```python
from build123d import *

# Parameters (mm, degrees)
RECORD_R             = 67.31
RECORD_R_2           = 1.054294776
RECORD_EXTRUDE_DEPTH = 2.54
MOTOR_HOLE_DEPTH     = 2.54


# Read off the part's stored shape, not the designer's step: Motor Hole
with BuildPart() as part:
    # Record → Record Extrude (new body)
    with BuildSketch(Plane(origin=(0, 0, 0), x_dir=(1, 0, 0), z_dir=(0, 1, 0))):
        with Locations(Location((13.743289035, -70.841587708, 0), (0, 0, 270))):
            Circle(RECORD_R)
        with Locations(Location((66.372058646, -74.952013208, 0), (0, 0, 270))):
            Circle(RECORD_R_2, mode=Mode.SUBTRACT)
        with Locations(Location((40.779568941, -74.952013208, 0), (0, 0, 270))):
            Circle(RECORD_R_2, mode=Mode.SUBTRACT)
    extrude(amount=RECORD_EXTRUDE_DEPTH)

    # Motor Hole outline → Motor Hole (cut)
    with BuildSketch(Plane(origin=(0, 0, 0), x_dir=(1, 0, 0), z_dir=(0, 1, 0))):
        with BuildLine():
            Line((11.872460342, -72.091587708), (15.614117728, -72.091587708))
            ThreePointArc((15.614117728, -72.091587708), (13.743289035, -68.591587708), (11.872460342, -72.091587708))
        make_face()
    extrude(amount=MOTOR_HOLE_DEPTH, mode=Mode.SUBTRACT)


solid = part.part
```
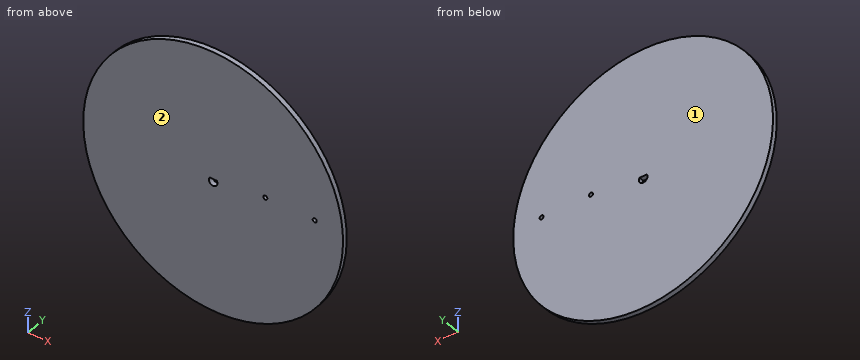
The model under review builds one solid part; all positions refer to its coordinate system, in mm. Face numbers are marked on the shaded views. Round coordinates to 2 decimals unless told otherwise and drop trailing zeros. Order: outer loops, then holes, each group sorted by start corner. A loop starts at its lowest first (then second) coordinate and runs counter-clockwise, first axis right, second up. Notation, with made-up numbers: (36.5, 51.5) -> (84.5, 51.5) arc R15 ccw to (84.5, 68.5) -> close; hole circle Ø8 at (87, 17). An arc over 180 degrees is marked (long way). One line per item, written item: value. Start each with the question number.
Q1. Mouldability with a two-part tool opening along Y and no side actions: class the marked faces 1 and 2 as released by +Y, released by -Y, zero draft, split by the parting line, or undercut.
Q2. Take a section at C-C (x = -43). Write out the cut boundary in (y, z), and give its area (3 significant figures).
Q3. Wall thickness on line 1 (Z direction, x = -31.5, y = 2.25); line 2 (Z direction, x = 56.5, y = 1.9); line 3 (X direction, y = 1.5, z = 30.5): over which ranges is each line inside the solid? List them lowest first.
Q4. Take a section at A-A (y = 0.4). Write out the cut boundary in (x, z).
Q5. Clearance check with flat-ended pins moving along their axes: pin 1 Ø1.9 at (x, z) = (66.37, 74.95) entering from -Y; pin 2 Ø1.5 at (y, z) = (1.5, 73) entering from -X; pin 3 Ø0.8 at (x, y) = (13, 1) entering from -Z. State where each tip first meets the part, or that it passes through.
Q6. Take a section at B-B (z = 49). Write out the cut boundary in (x, y), and give its area (3 significant figures).
Reported:
1. face 1: released by +Y
1. face 2: released by -Y
2. outline: (0, 34.64) -> (2.54, 34.64) -> (2.54, 107.05) -> (0, 107.05) -> close
2. area: 184 mm2
3. line 1: z = 21.01 to 120.68
3. line 2: z = 18.86 to 122.83
3. line 3: x = -40.14 to 67.62
4. outline: circle Ø134.62 at (13.74, 70.84); hole (11.87, 72.09) arc R2.25 ccw (long way) to (15.61, 72.09) -> close; hole circle Ø2.11 at (40.78, 74.95); hole circle Ø2.11 at (66.37, 74.95)
5. pin 1: passes through
5. pin 2: stops at x = -53.55
5. pin 3: stops at z = 3.53
6. outline: (-49.92, 0) -> (77.41, 0) -> (77.41, 2.54) -> (-49.92, 2.54) -> close
6. area: 323 mm2
